Geometry: final body of the model. Coordinates: model frame, mm. A direction names the side the tool comes from. Round coordinates to 2 decimals unless told otherwise and drop trailing zeros. Write each loop counter-clockwise with the first axis right and the second up, starting at its lowest first coordinate (ties: lowest second). Pieces come first, ordered by that corner, then holes. Notation, with made-up numbers: (66, 26.25) -> (118, 26.25) arc R4 cw to (118, 33.25) -> close; hole circle Ø7 at (-29, -40). An arc over 180 degrees is marked (long way). One line per item, written item: value. Start each with the question number.
from build123d import *

# Parameters (mm, degrees)
SKETCH_1_W               = 57
SKETCH_1_H               = 57
EXTRUDE_1_DEPTH          = 99
CUT_EXTRUDE_1_DEPTH      = 90
SKETCH_3_R               = 4
EXTRUDE_2_DEPTH          = 21
PATTERN_CIRCULAR_1_COUNT = 4
SKETCH_5_R               = 19
EXTRUDE_3_DEPTH          = 1.6


with BuildPart() as part:
    # Sketch 1 → Extrude 1 (new body)
    with BuildSketch(Plane(origin=(0, 0, 0), x_dir=(1, 0, 0), z_dir=(0, 1, 0))):
        Rectangle(SKETCH_1_W, SKETCH_1_H)
    extrude(amount=EXTRUDE_1_DEPTH)

    # Sketch 2 → Cut-Extrude 1 (cut)
    with BuildSketch(Plane.XZ):
        with BuildLine():
            Line((28.5, -28.5), (28.5, -22.5))
            ThreePointArc((28.5, -22.5), (24.257359313, -24.257359313), (22.5, -28.5))
            Line((22.5, -28.5), (28.5, -28.5))
        make_face()
    cut_extrude_1 = extrude(amount=-CUT_EXTRUDE_1_DEPTH, mode=Mode.SUBTRACT)

    # Sketch 3 → Extrude 2 (add)
    with BuildSketch(Plane(origin=(0, 99, 0), x_dir=(1, 0, 0), z_dir=(0, 1, 0))):
        with Locations(Location((0, 0, 0), (0, 0, 90))):
            Circle(SKETCH_3_R)
    extrude(amount=EXTRUDE_2_DEPTH)

    # Pattern Circular 1: Cut-Extrude 1 ×4 about axis
    pattern_circular_1_axis = Axis((0, 0, 0), (0, 1, 0))
    for i in range(1, PATTERN_CIRCULAR_1_COUNT):
        add(cut_extrude_1.rotate(pattern_circular_1_axis, i * 360 / PATTERN_CIRCULAR_1_COUNT), mode=Mode.SUBTRACT)

    # Sketch 5 → Extrude 3 (add)
    with BuildSketch(Plane(origin=(0, 99, 0), x_dir=(1, 0, 0), z_dir=(0, 1, 0))):
        with Locations(Location((0, 0, 0), (0, 0, 90))):
            Circle(SKETCH_5_R)
    extrude(amount=EXTRUDE_3_DEPTH)


solid = part.part
(1) Line query: probe 1 along Y at (x, z) = (-11, -12.5); probe 2 along Y at (x, z) = (-13.5, -16); probe 3 along X at (y, z) = (12.5, -25). Output: solid intervals per line, ascending.
(2) Section query B-B (x = 0). Output: boundary loops of the cut face in (y, z).
(3) Section query C-C (z = 0). Output: boundary loops of the cut face in (x, y), and give its area (3 significant figures).
(4) Set-up query: faces 1 (the face through (-24.211, 44.37, -24.304)), 2 (the face through (-24.304, 44.37, 24.211)), 3 (the face through (-0.4, 99, -19.4)), 4 (the face through (24.211, 44.37, 24.304)). Return all of +Z, -Z, +X, -X, +Y, -Y with unobstructed straight access to the full face (end or side cutting, diameter ignored); none if empty.
(5) Section query D-D (z = 15). Output: boundary loops of the cut face in (x, y), and give its area (3 significant figures).
(6) Pin query (flat end, axial travel): pin 1 (1.8 mm diameter, centred on x = 25, z = -26.5, fed in from -Y); pin 2 (6 mm diameter, centred on x = -6, z = -7.5, fed in from +Y). Return the tip coordinate at first contact, or that it passes through.
(7) Section query A-A (y = 28.5). Output: boundary loops of the cut face in (x, z), and give its area (3 significant figures).
Results list:
1. probe 1: y = 0 to 100.6
1. probe 2: y = 0 to 99
1. probe 3: x = -23.63 to 23.63
2. outline: (0, -28.5) -> (99, -28.5) -> (99, -19) -> (100.6, -19) -> (100.6, -4) -> (120, -4) -> (120, 4) -> (100.6, 4) -> (100.6, 19) -> (99, 19) -> (99, 28.5) -> (0, 28.5) -> close
3. outline: (-28.5, 0) -> (28.5, 0) -> (28.5, 99) -> (19, 99) -> (19, 100.6) -> (4, 100.6) -> (4, 120) -> (-4, 120) -> (-4, 100.6) -> (-19, 100.6) -> (-19, 99) -> (-28.5, 99) -> close
3. area: 5,860 mm^2
4. face 1: -Z, -X, -Y
4. face 2: +Z, -X, -Y
4. face 3: +Y
4. face 4: +Z, +X, -Y
5. outline: (-28.5, 0) -> (28.5, 0) -> (28.5, 99) -> (11.66, 99) -> (11.66, 100.6) -> (-11.66, 100.6) -> (-11.66, 99) -> (-28.5, 99) -> close
5. area: 5,680 mm^2
6. pin 1: stops at y = 90
6. pin 2: stops at y = 100.6
7. outline: (-28.5, -22.5) arc R6 cw to (-22.5, -28.5) -> (22.5, -28.5) arc R6 cw to (28.5, -22.5) -> (28.5, 22.5) arc R6 cw to (22.5, 28.5) -> (-22.5, 28.5) arc R6 cw to (-28.5, 22.5) -> close
7. area: 3,140 mm^2
